from build123d import *

# Parameters (mm, degrees)
SKETCH_1_W             = 34
SKETCH_1_H             = 34
EXTRUDE_1_DEPTH        = 1.5
SKETCH_2_R             = 2.5
SKETCH_2_R_2           = 1.55
CUT_EXTRUDE_1_DEPTH    = 49.106652347
SKETCH_3_R             = 1.25
CUT_EXTRUDE_2_DEPTH    = 49.106652347
CUT_EXTRUDE_3_DEPTH    = 49.106652347
FILLET_1_R             = 1.25
FILLET_1_OF_MIRROR_3_R = 1.25
FILLET_2_R             = 3


with BuildPart() as part:
    # ｽｹｯﾁ1 → ﾎﾞｽ - 押し出し1 (new body)
    with BuildSketch(Plane.XY):
        with Locations((17, 17)):
            Rectangle(SKETCH_1_W, SKETCH_1_H)
    extrude(amount=EXTRUDE_1_DEPTH)

    # ｽｹｯﾁ2 → ｶｯﾄ - 押し出し1 (cut, through all)
    with BuildSketch(Plane.XY.offset(1.5)):
        with Locations((17, 17)):
            Circle(SKETCH_2_R)
        with Locations((3, 31)):
            Circle(SKETCH_2_R_2)
        with Locations((31, 31)):
            Circle(SKETCH_2_R_2)
        with Locations((3, 3)):
            Circle(SKETCH_2_R_2)
        with Locations((31, 3)):
            Circle(SKETCH_2_R_2)
    extrude(amount=-CUT_EXTRUDE_1_DEPTH, mode=Mode.SUBTRACT)

    # ｽｹｯﾁ3 → ｶｯﾄ - 押し出し2 (cut, through all)
    with BuildSketch(Plane.XY.offset(1.5)):
        with BuildLine():
            Line((2.5, 22), (2.5, 13.25))
            ThreePointArc((2.5, 13.25), (3.75, 14.5), (5, 13.25))
            Line((5, 13.25), (5, 21))
            ThreePointArc((5, 21), (7.196699141, 26.303300859), (12.5, 28.5))
            Line((12.5, 28.5), (17, 28.5))
            Line((17, 28.5), (17, 31))
            Line((17, 31), (11.5, 31))
            ThreePointArc((11.5, 31), (5.136038969, 28.363961031), (2.5, 22))
        make_face()
        with Locations((3.75, 13.25)):
            Circle(SKETCH_3_R)
    cut_extrude_2 = extrude(amount=-CUT_EXTRUDE_2_DEPTH, mode=Mode.SUBTRACT)

    # ﾐﾗｰ1: ｶｯﾄ - 押し出し2 across plane
    add(cut_extrude_2.mirror(Plane(origin=(17, 0, 0), x_dir=(0, 0, 1), z_dir=(1, 0, 0))), mode=Mode.SUBTRACT)

    # ｽｹｯﾁ4 → ｶｯﾄ - 押し出し3 (cut, through all)
    with BuildSketch(Plane.XY.offset(1.5)):
        with BuildLine():
            ThreePointArc((17, 12), (13.464466094, 13.464466094), (12, 17))
            Line((12, 17), (12, 22))
            Line((12, 22), (9.5, 22))
            Line((9.5, 22), (9.5, 16.5))
            ThreePointArc((9.5, 16.5), (11.550252532, 11.550252532), (16.5, 9.5))
            Line((16.5, 9.5), (17, 9.5))
            Line((17, 9.5), (17, 12))
        make_face()
    cut_extrude_3 = extrude(amount=-CUT_EXTRUDE_3_DEPTH, mode=Mode.SUBTRACT)

    # ﾌｨﾚｯﾄ1
    fillet_1_edges = [part.edges().sort_by_distance(p)[0] for p in [
        (12, 22, 0.75),
        (9.5, 22, 0.75),
    ]]
    fillet(fillet_1_edges, radius=FILLET_1_R - 0.0001)  # a hair under: the kernel refuses the full size

    # ﾐﾗｰ3: ｶｯﾄ - 押し出し3 across plane
    add(cut_extrude_3.mirror(Plane(origin=(17, 0, 0), x_dir=(0, 0, 1), z_dir=(1, 0, 0))), mode=Mode.SUBTRACT)

    # ﾌｨﾚｯﾄ1 of ﾐﾗｰ3
    fillet_1_of_mirror_3_edges = [part.edges().sort_by_distance(p)[0] for p in [
        (22, 22, 0.75),
        (24.5, 22, 0.75),
    ]]
    fillet(fillet_1_of_mirror_3_edges, radius=FILLET_1_OF_MIRROR_3_R - 0.0001)  # a hair under: the kernel refuses the full size

    # ﾌｨﾚｯﾄ2
    fillet_2_edges = [part.edges().sort_by_distance(p)[0] for p in [
        (0, 34, 0.75),
        (34, 34, 0.75),
        (34, 0, 0.75),
        (0, 0, 0.75),
    ]]
    fillet(fillet_2_edges, radius=FILLET_2_R)


solid = part.part
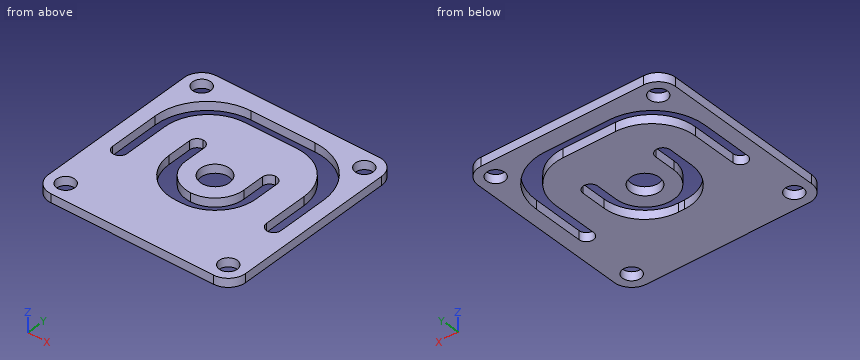
Source: CAD feature listing. Evaluate the final solid. Frame: model axes, mm. Round coordinates to 2 decimals unless told otherwise and drop trailing zeros. Loops run counter-clockwise (first coordinate to the right, second up) from the corner with the lowest first, then second, coordinate; pieces in that order, holes last.
Q1. Section A-A, the plane x = 8. Return loops of the section in (y, z), plus the area to 3 significant figures.
Q2. First-contact query: P1, Ø2.5, axis at x = 31, y = 3, coming from the +Z side. Flat tip, straight axial feed; report the tip coordinate or a pass-through.
Q3. Ray query, line 1 (Y direction, x = 32, z = 0.6); line 2 (X direction, y = 13, z = 0.3); line 3 (Y direction, x = 13.5, z = 0.9). Return the intervals inside material, ascending.
Q4. Section B-B, the plane x = 3.75. Return loops of the section in (y, z).
Q5. Section C-C, the plane z = 0.9. State how many separate pieces and enclosed holes the cut face has, plus the area to 3 significant figures.
Q6. Section D-D, the plane x = 26.5. Return loops of the section in (y, z), plus the area to 3 significant figures.
Solutions:
1. outline: (0, 0) - (27, 0) - (27, 1.5) - (0, 1.5) - close; (30.29, 0) - (34, 0) - (34, 1.5) - (30.29, 1.5) - close
1. area: 46.1 mm2
2. P1: passes through
3. line 1: y = 0.17 to 1.82, 4.18 to 29.82, 32.18 to 33.83
3. line 2: x = 0 to 2.53, 4.97 to 10.44, 14 to 20, 23.56 to 29.03, 31.47 to 34
3. line 3: y = 0 to 10.18, 13.43 to 28.5, 31 to 34
4. outline: (0, 0) - (1.64, 0) - (1.64, 1.5) - (0, 1.5) - close; (4.36, 0) - (12, 0) - (12, 1.5) - (4.36, 1.5) - close; (26.58, 0) - (29.64, 0) - (29.64, 1.5) - (26.58, 1.5) - close; (32.36, 0) - (34, 0) - (34, 1.5) - (32.36, 1.5) - close
5. separate pieces: 1
5. enclosed holes: 7
5. area: 880 mm2
6. outline: (0, 0) - (26.59, 0) - (26.59, 1.5) - (0, 1.5) - close; (30.06, 0) - (34, 0) - (34, 1.5) - (30.06, 1.5) - close
6. area: 45.8 mm2
